```python
from build123d import *

# Parameters (mm, degrees)
ESBO_O1_R                = 2.4
ESBO_O1_W                = 30
ESBO_O1_H                = 4
RESSALTO_EXTRUS_O1_DEPTH = 4
ESBO_O3_R                = 4
CORTE_EXTRUS_O1_DEPTH    = 6
FURO_COM_FOLGA_DE_M41_D  = 4.5
ESBO_O7_W                = 60
ESBO_O7_H                = 2
CORTE_EXTRUS_O4_DEPTH    = 5
RESSALTO_EXTRUS_O2_DEPTH = 4


with BuildPart() as part:
    # Esboço1 → Ressalto-extrusão1 (new body)
    with BuildSketch(Plane.XY):
        with BuildLine():
            Line((0, 0), (400, 0))
            Line((400, 0), (400, 140))
            ThreePointArc((400, 140), (397.071067812, 147.071067812), (390, 150))
            Line((390, 150), (130, 150))
            ThreePointArc((130, 150), (122.928932188, 147.071067812), (120, 140))
            Line((120, 140), (120, 130))
            Line((120, 130), (60, 130))
            Line((60, 130), (60, 140))
            ThreePointArc((60, 140), (57.071067812, 147.071067812), (50, 150))
            Line((50, 150), (10, 150))
            ThreePointArc((10, 150), (2.928932188, 147.071067812), (0, 140))
            Line((0, 140), (0, 0))
        make_face()
        with Locations((30, 133.5)):
            Circle(ESBO_O1_R, mode=Mode.SUBTRACT)
        with Locations((30, 96.5)):
            Circle(ESBO_O1_R, mode=Mode.SUBTRACT)
        with Locations((100, 126)):
            Rectangle(ESBO_O1_W, ESBO_O1_H, mode=Mode.SUBTRACT)
        with Locations((200, 126)):
            Rectangle(ESBO_O1_W, ESBO_O1_H, mode=Mode.SUBTRACT)
        with Locations((300, 126)):
            Rectangle(ESBO_O1_W, ESBO_O1_H, mode=Mode.SUBTRACT)
        with BuildLine():
            Line((365, 135.9), (375, 135.9))
            ThreePointArc((375, 135.9), (377.4, 133.5), (375, 131.1))
            Line((375, 131.1), (365, 131.1))
            ThreePointArc((365, 131.1), (362.6, 133.5), (365, 135.9))
        make_face(mode=Mode.SUBTRACT)
        with BuildLine():
            Line((365, 98.9), (375, 98.9))
            ThreePointArc((375, 98.9), (377.4, 96.5), (375, 94.1))
            Line((375, 94.1), (365, 94.1))
            ThreePointArc((365, 94.1), (362.6, 96.5), (365, 98.9))
        make_face(mode=Mode.SUBTRACT)
    extrude(amount=RESSALTO_EXTRUS_O1_DEPTH)

    # Esboço3 → Corte-extrusão1 (cut)
    with BuildSketch(Plane.XY.offset(4)):
        with Locations((30, 115)):
            Circle(ESBO_O3_R)
        with BuildLine():
            Line((365, 119), (375, 119))
            ThreePointArc((375, 119), (379, 115), (375, 111))
            Line((375, 111), (365, 111))
            ThreePointArc((365, 111), (361, 115), (365, 119))
        make_face()
    extrude(amount=-CORTE_EXTRUS_O1_DEPTH, mode=Mode.SUBTRACT)

    # Furo com folga de M41 (through all)
    with Locations(Plane(origin=(350, 12.5, 4), x_dir=(1, 0, 0), z_dir=(0, 0, 1))):
        with Locations((0, 0), (-225, 62.5), (-75, 62.5), (-300, 0), (-200, 0), (-100, 0)):
            Hole(FURO_COM_FOLGA_DE_M41_D / 2)

    # Esboço7 → Corte-extrusão4 (cut, through all)
    with BuildSketch(Plane.XY.offset(4)):
        with Locations((90, 129)):
            Rectangle(ESBO_O7_W, ESBO_O7_H)
    extrude(amount=-CORTE_EXTRUS_O4_DEPTH, mode=Mode.SUBTRACT)

    # Esboço8 → Ressalto-extrusão2 (add)
    with BuildSketch(Plane.XY.offset(4)):
        with BuildLine():
            Line((10, 158), (50, 158))
            ThreePointArc((50, 158), (57.071067812, 155.071067812), (60, 148))
            Line((60, 148), (60, 140))
            ThreePointArc((60, 140), (57.071067812, 147.071067812), (50, 150))
            Line((50, 150), (10, 150))
            ThreePointArc((10, 150), (2.928932188, 147.071067812), (0, 140))
            Line((0, 140), (0, 148))
            ThreePointArc((0, 148), (2.928932188, 155.071067812), (10, 158))
        make_face()
        with BuildLine():
            Line((120, 140), (120, 148))
            ThreePointArc((120, 148), (122.928932188, 155.071067812), (130, 158))
            Line((130, 158), (390, 158))
            ThreePointArc((390, 158), (397.071067812, 155.071067812), (400, 148))
            Line((400, 148), (400, 140))
            ThreePointArc((400, 140), (397.071067812, 147.071067812), (390, 150))
            Line((390, 150), (130, 150))
            ThreePointArc((130, 150), (122.928932188, 147.071067812), (120, 140))
        make_face()
    extrude(amount=-RESSALTO_EXTRUS_O2_DEPTH)


solid = part.part
```
The model under review builds one solid part; all positions refer to its coordinate system, in mm. A direction names the side the tool comes from. Round coordinates to 2 decimals unless told otherwise and drop trailing zeros. Loops run counter-clockwise (first coordinate to the right, second up) from the corner with the lowest first, then second, coordinate; pieces in that order, holes last. Notation, with made-up numbers: (3, -17.75) -> (27, -17.75) arc R7 cw to (27, -5.75) -> close; hole circle Ø1 at (84, -16). An arc over 180 degrees is marked (long way). Answer in a Markdown table with one row per item.
1) Consider section A-A, the plane y = 115. Write out the cut boundary in (x, z).
Taken from the geometry:
| item | result |
|---|---|
| outline | (0, 0) -> (26, 0) -> (26, 4) -> (0, 4) -> close; (34, 0) -> (361, 0) -> (361, 4) -> (34, 4) -> close; (379, 0) -> (400, 0) -> (400, 4) -> (379, 4) -> close |
2) Tool access review of faces 4 (the cylindrical face through (29.479, 118.966, 2.028)), 5 (the cylindrical face through (56.99, 155.15, 2.03)): name each direction out of +Z, -Z, +X, -X, +Y, -Y from which nothing blocks a thin tool from reaching the whole face with its end or side.
Taken from the geometry:
| item | result |
|---|---|
| face 4 | +Z, -Z |
| face 5 | +Z, -Z, +Y |
3) Consider section B-B, the plane x = 210. Write out the cut boundary in (y, z).
Taken from the geometry:
| item | result |
|---|---|
| outline | (0, 0) -> (124, 0) -> (124, 4) -> (0, 4) -> close; (128, 0) -> (158, 0) -> (158, 4) -> (128, 4) -> close |
4) Consider section C-C, the plane z = 1.15. Count the separate pieces of the cut face and the enclosed holes in it, plus the area to 3 significant figures.
Taken from the geometry:
| item | result |
|---|---|
| separate pieces | 1 |
| enclosed holes | 14 |
| area | 60,500 mm² |
5) Wall thickness on line 1 along Y through (x, z) = (30, 2.95); line 2 along Y through (x, z) = (30.5, 1.9); line 3 along X through (y, z) = (113, 1.4): over which ranges is each line inside the solid? List them lowest first.
Taken from the geometry:
| item | result |
|---|---|
| line 1 | y = 0 to 94.1, 98.9 to 111, 119 to 131.1, 135.9 to 158 |
| line 2 | y = 0 to 94.15, 98.85 to 111.03, 118.97 to 131.15, 135.85 to 158 |
| line 3 | x = 0 to 26.54, 33.46 to 361.54, 378.46 to 400 |
6) For pin 1 Ø2.5 at (x, y) = (250, 12.5) entering from +Z; pin 2 Ø6 at (x, y) = (343.5, 69) entering from -Z; pin 3 Ø2 at (x, z) = (102.5, 2.5) entering from +Y, all flat-tipped, find the tip position at first contact; note any pin that passes through.
Taken from the geometry:
| item | result |
|---|---|
| pin 1 | passes through |
| pin 2 | stops at z = 0 |
| pin 3 | stops at y = 124 |
7) Draft analysis for pull direction X (two halves, no side actions). For faces 1 (the cylindrical face through (396.99, 155.15, 2.03)), 2 (the cylindrical face through (122.85, 154.99, 2.03)), 3 (the flat face through (203, 80, 0)), state which applies: pulls with the +X half, pulls with the -X half, needs draft (parallel to the pull), parting line crosses it, or undercut.
Taken from the geometry:
| item | result |
|---|---|
| face 1 | pulls with the +X half |
| face 2 | undercut |
| face 3 | needs draft |
